from build123d import *

# Parameters (mm, degrees)
SKETCH1_R           = 7
SKETCH1_R_2         = 4
BOSS_EXTRUDE1_DEPTH = 13
SKETCH5_W           = 17
SKETCH5_H           = 16
BOSS_EXTRUDE3_DEPTH = 3
CUT_EXTRUDE2_START  = -14
SKETCH7_R           = 4
CUT_EXTRUDE2_DEPTH  = 14
SKETCH6_W           = 17
SKETCH6_H           = 16
BOSS_EXTRUDE5_DEPTH = 10


with BuildPart() as part:
    # Sketch1 → Boss-Extrude1 (new body)
    with BuildSketch(Plane(origin=(0, 0, 0), x_dir=(1, 0, 0), z_dir=(0, 1, 0))):
        with Locations(Location((0, 0, 0), (0, 0, 90))):
            Circle(SKETCH1_R)
        with Locations(Location((0, 0, 0), (0, 0, 90))):
            Circle(SKETCH1_R_2, mode=Mode.SUBTRACT)
    extrude(amount=BOSS_EXTRUDE1_DEPTH)

    # Sketch5 → Boss-Extrude3 (add)
    with BuildSketch(Plane(origin=(0, 10, 0), x_dir=(1, 0, 0), z_dir=(0, 1, 0))):
        Rectangle(SKETCH5_W, SKETCH5_H)
    extrude(amount=BOSS_EXTRUDE3_DEPTH)

    # Sketch7 → Cut-Extrude2 (cut)
    with BuildSketch(Plane(origin=(0, 13, 0), x_dir=(1, 0, 0), z_dir=(0, 1, 0)).offset(CUT_EXTRUDE2_START)):
        with Locations(Location((0, 0, 0), (0, 0, 90))):
            Circle(SKETCH7_R)
    extrude(amount=CUT_EXTRUDE2_DEPTH, mode=Mode.SUBTRACT)

    # Sketch6 → Boss-Extrude5 (add)
    with BuildSketch(Plane(origin=(0, 13, 0), x_dir=(1, 0, 0), z_dir=(0, 1, 0))):
        Rectangle(SKETCH6_W, SKETCH6_H)
        with BuildLine():
            ThreePointArc((2.783882181, -7.5), (8, 0), (2.783882181, 7.5))
            Line((2.783882181, 7.5), (-2.783882181, 7.5))
            ThreePointArc((-2.783882181, 7.5), (-8, 0), (-2.783882181, -7.5))
            Line((-2.783882181, -7.5), (2.783882181, -7.5))
        make_face(mode=Mode.SUBTRACT)
    extrude(amount=BOSS_EXTRUDE5_DEPTH)


solid = part.part
Verification items for the finished model (mm, model axes). A direction names the side the tool comes from. Round coordinates to 2 decimals unless told otherwise and drop trailing zeros. Write each loop counter-clockwise with the first axis right and the second up, starting at its lowest first coordinate (ties: lowest second). Pieces come first, ordered by that corner, then holes.
(1) Depth check by flat-ended pin: pin 1 Ø2 at (x, z) = (2.5, 3) entering from +Y; pin 2 Ø4 at (y, z) = (7.5, 5.5) entering from -X. Enter the tip coordinate at first touch or a pass-through.
Returned:
pin 1: stops at y = 13
pin 2: stops at x = -6.06
(2) Section check D-D (x = -6.5). Enter the section's corners in (y, z).
Returned:
outline: (0, -2.6) - (10, -2.6) - (10, -8) - (23, -8) - (23, -4.66) - (13, -4.66) - (13, 4.66) - (23, 4.66) - (23, 8) - (10, 8) - (10, 2.6) - (0, 2.6) - close
(3) Mould release check, pull along X, two halves, no side actions. Record for faces 4 (the flat face through (0, 18, 7.5)), 5 (the flat face through (8.5, 16, 0)), 6 (the flat face through (0, 16, 8)): pulls with the +X half, pulls with the -X half, needs draft (parallel to the pull), parting line crosses it, or undercut.
Returned:
face 4: undercut
face 5: pulls with the +X half
face 6: needs draft
(4) Material ranges on line 1 (X direction, y = 9.75, z = 0); line 2 (Z direction, x = -1, y = 18.25); line 3 (Y direction, x = 7.5, z = 3.5), recorded low to high.
Returned:
line 1: x = -7 to -4, 4 to 7
line 2: z = -8 to -7.5, 7.5 to 8
line 3: y = 10 to 23
(5) Section check B-B (y = 18.5). Enter the section's corners in (x, z).
Returned:
outline: (-8.5, -8) - (8.5, -8) - (8.5, 8) - (-8.5, 8) - close; hole (-2.78, -7.5) - (2.78, -7.5) arc R8 ccw to (2.78, 7.5) - (-2.78, 7.5) arc R8 ccw to start
(6) Access from +Z, -Z, +X, -X, +Y, -Y to the whole of each face (thin tool, end or side, straight path). Record for faces 1 (the cylindrical face through (8, 18, 0)), 2 (the flat face through (-0.1, 10, -7.2)), 3 (the flat face through (0, 16, -8)).
Returned:
face 1: +Y
face 2: -Y
face 3: -Z, +X, -X, +Y, -Y
(7) Section check C-C (x = 0). Enter the section's corners in (y, z), plus the area to 3 significant figures.
Returned:
outline: (0, -7) - (10, -7) - (10, -8) - (23, -8) - (23, -7.5) - (13, -7.5) - (13, -4) - (0, -4) - close; (0, 4) - (13, 4) - (13, 7.5) - (23, 7.5) - (23, 8) - (10, 8) - (10, 7) - (0, 7) - close
area: 94.0 mm2
(8) Section check A-A (z = 0). Enter the section's corners in (x, y), plus the area to 3 significant figures.
Returned:
outline: (-8.5, 10) - (-7, 10) - (-7, 0) - (-4, 0) - (-4, 13) - (-8, 13) - (-8, 23) - (-8.5, 23) - close; (4, 0) - (7, 0) - (7, 10) - (8.5, 10) - (8.5, 23) - (8, 23) - (8, 13) - (4, 13) - close
area: 97.0 mm2
